```python
from build123d import *

# Parameters (mm, degrees)
SKETCH1_W               = 120
SKETCH1_H               = 220
BOSS_EXTRUDE1_DEPTH     = 50
SKETCH2_W               = 140
SKETCH2_H               = 240
BOSS_EXTRUDE2_DEPTH     = 1.5
SHELL1_T                = 2
CUT_EXTRUDE1_DEPTH      = 183.855817518
CUT_EXTRUDE1_DEPTH_BACK = 183.855817518
FILLET1_R               = 2
FILLET2_R               = 2
SKETCH9_R               = 4.951117386
CUT_EXTRUDE2_DEPTH      = 149.162917088
F_1_5MM_DOWEL_HOLE1_D   = 1.5


with BuildPart() as part:
    # Sketch1 → Boss-Extrude1 (new body)
    with BuildSketch(Plane.XY):
        Rectangle(SKETCH1_W, SKETCH1_H)
    extrude(amount=BOSS_EXTRUDE1_DEPTH)

    # Sketch2 → Boss-Extrude2 (add)
    with BuildSketch(Plane.XY.offset(50)):
        Rectangle(SKETCH2_W, SKETCH2_H)
    extrude(amount=BOSS_EXTRUDE2_DEPTH)

    # Shell1
    # the kernel refuses this shell: the inside is offset whole and opened at the faces by hand
    shell1_offset = offset(amount=-SHELL1_T, mode=Mode.PRIVATE)
    shell1_offset = shell1_offset + extrude(shell1_offset.faces().sort_by_distance((0, 0, 49.5))[0], amount=SHELL1_T, mode=Mode.PRIVATE)
    add(shell1_offset, mode=Mode.SUBTRACT)

    # Sketch8 → Cut-Extrude1 (cut, two sides: drawn at the far end of the back side and taken through both)
    with BuildSketch(Plane.ZY.offset(-58).offset(-CUT_EXTRUDE1_DEPTH_BACK)):
        with BuildLine():
            Line((51.5, -83), (44.5, -83))
            ThreePointArc((44.5, -83), (41, -86.5), (44.5, -90))
            Line((44.5, -90), (51.5, -90))
            Line((51.5, -90), (51.5, -83))
        make_face()
    extrude(amount=CUT_EXTRUDE1_DEPTH + CUT_EXTRUDE1_DEPTH_BACK, mode=Mode.SUBTRACT)

    # Fillet1
    fillet1_edges = [part.edges().sort_by_distance(p)[0] for p in [
        (0, -108, 2),
        (-60, 0, 0),
        (0, 110, 0),
        (60, 0, 0),
    ]]
    fillet(fillet1_edges, radius=FILLET1_R)

    # Fillet2
    # the kernel refuses this fillet: 2 mm, written as the material it adds along each edge
    with BuildSketch(Plane(origin=(58, 108, 51.5), x_dir=(0, -1, 0), z_dir=(0, 0, -1))) as fillet2_piece_1:
        with BuildLine():
            CenterArc((FILLET2_R, FILLET2_R), FILLET2_R, 180, 90)
            Line((0, FILLET2_R), (0, 0))
            Line((0, 0), (FILLET2_R, 0))
        make_face()
    extrude(amount=49.5)
    # the kernel refuses this fillet: 2 mm, written as the material it takes off along each edge
    with BuildSketch(Plane(origin=(-58, 108, 2), x_dir=(0, 1, 0), z_dir=(-1, 0, 0))) as fillet2_2_piece_1_section:
        Polygon((0, 0), (FILLET2_R * 1.02, 0), (FILLET2_R * 1.02, FILLET2_R * 1.02), (0, FILLET2_R * 1.02), align=None)
    fillet2_2_piece_1 = extrude(amount=FILLET2_R * 1.02, mode=Mode.PRIVATE)
    fillet2_2_piece_1 = fillet2_2_piece_1 - Plane(origin=(-58, 108, 2), x_dir=(0, -0.7071067811865475, 0.7071067811865475), z_dir=(-1, 0, 0)) * Sphere(FILLET2_R, mode=Mode.PRIVATE)
    add(fillet2_2_piece_1, mode=Mode.SUBTRACT)
    with BuildSketch(Plane(origin=(60, -110, 2), x_dir=(-1, 0, 0), z_dir=(0, 0, 1)), Plane(origin=(-60, -110, 2), x_dir=(0, 1, 0), z_dir=(0, 0, 1))) as fillet2_2_piece_2:
        with BuildLine():
            CenterArc((FILLET2_R, -FILLET2_R), FILLET2_R, 90, 90)
            Line((0, -FILLET2_R), (0, 0))
            Line((0, 0), (FILLET2_R, 0))
        make_face()
    extrude(amount=48, mode=Mode.SUBTRACT)
    with BuildSketch(Plane(origin=(-60, 110, 2), x_dir=(0, -1, 0), z_dir=(0, 0, 1))) as fillet2_2_piece_3:
        with BuildLine():
            CenterArc((FILLET2_R, FILLET2_R), FILLET2_R, 180, 90)
            Line((0, FILLET2_R), (0, 0))
            Line((0, 0), (FILLET2_R, 0))
        make_face()
    extrude(amount=48, mode=Mode.SUBTRACT)
    with BuildSketch(Plane(origin=(58, -110, 0), x_dir=(0, 0, 1), z_dir=(-1, 0, 0))) as fillet2_2_piece_4:
        with BuildLine():
            CenterArc((FILLET2_R, FILLET2_R), FILLET2_R, 180, 90)
            Line((0, FILLET2_R), (0, 0))
            Line((0, 0), (FILLET2_R, 0))
        make_face()
    extrude(amount=116, mode=Mode.SUBTRACT)
    with BuildSketch(Plane(origin=(58, -110, 2), x_dir=(1, 0, 0), z_dir=(0, 0, 1))) as fillet2_2_piece_5:
        with BuildLine():
            CenterArc((2 - FILLET2_R, FILLET2_R), FILLET2_R, 270, 90)
            Line((2, FILLET2_R), (2, 0))
            Line((2, 0), (2 - FILLET2_R, 0))
        make_face()
    revolve(axis=Axis((58, -110, 2), (0, 1, 0)), revolution_arc=90, mode=Mode.SUBTRACT)
    with BuildSketch(Plane(origin=(-58, -110, 2), x_dir=(-1, 0, 0), z_dir=(0, 0, 1))) as fillet2_2_piece_6:
        with BuildLine():
            CenterArc((2 - FILLET2_R, -FILLET2_R), FILLET2_R, 0, 90)
            Line((2 - FILLET2_R, 0), (2, 0))
            Line((2, 0), (2, -FILLET2_R))
        make_face()
    revolve(axis=Axis((-58, -110, 2), (0, -1, 0)), revolution_arc=90, mode=Mode.SUBTRACT)

    # Sketch9 → Cut-Extrude2 (cut, through all)
    with BuildSketch(Plane(origin=(0, 0, 0), x_dir=(-1, 0, 0), z_dir=(0, 0, -1))):
        with Locations((0, -88)):
            Circle(SKETCH9_R)
    extrude(amount=-CUT_EXTRUDE2_DEPTH, mode=Mode.SUBTRACT)

    # Ø1.5mm Dowel Hole1 (through all)
    with Locations(Plane(origin=(-164.627139737, -264.125226739, 50), x_dir=(-1, 0, 0), z_dir=(0, 0, -1))):
        with Locations((-229.627139737, 379.125226739), (-99.627139737, 379.125226739), (-229.627139737, 149.125226739), (-99.627139737, 149.125226739)):
            Hole(F_1_5MM_DOWEL_HOLE1_D / 2)


solid = part.part
```
Geometry check sheet. Reference: the model listing, model coordinates, mm. A direction names the side the tool comes from. Round coordinates to 2 decimals unless told otherwise and drop trailing zeros. Loops run counter-clockwise (first coordinate to the right, second up) from the corner with the lowest first, then second, coordinate; pieces in that order, holes last. Notation, with made-up numbers: (49.5, -38.5) - (64.5, -38.5) arc R15 ccw to (64.5, -27.5) - close; hole circle Ø1 at (48.5, 44.5). An arc over 180 degrees is marked (long way). Write each question's results on one line, items separated by ' | '. Start each with the question number.
Q1. Access from +Z, -Z, +X, -X, +Y, -Y to the whole of each face (thin tool, end or side, straight path). Record for faces 4 (the flat face through (-1, -110, 26)), 5 (the flat face through (-60, -2, 26)), 6 (the flat face through (-63, 34, 50)).
Q2. Cross-section at A-A on x = 0. Enter the section's corners in (y, z), and give its area (3 significant figures).
Q3. Thickness scan on line 1 (X direction, y = -115, z = 50.55); line 2 (Y direction, x = 65, z = 50.65); line 3 (X direction, y = -6, z = 32). Record the ranges inside material, lowest first. Write a range as [from, to].
Q4. Cross-section at B-B on z = 47. Enter the section's corners in (x, y), and give its area (3 significant figures).
Q5. Cross-section at D-D on y = 58. Enter the section's corners in (x, z).
Q6. Cross-section at C-C on z = 15. Enter the section's corners in (x, y), and give its area (3 significant figures).
Q7. Gauge pin test, flat ends, axial feed: P1, Ø2, axis at x = 65, y = 115, coming from the -Z side; P2, Ø10, axis at x = 40.5, z = 29.5, coming from the -Y side; P3, Ø1, axis at x = -55, y = 6, coming from the +Z side; P4, Ø0.9, axis at x = -65, y = 115, coming from the -Z side. Record the tip position at first contact, or that the pin passes through.
Q8. Release check for a two-part mould opening along X. For faces 1 (the flat face through (60, -1, 26)), 2 (the flat face through (-1, -108, 27)), 3 (the flat face through (62, 41, 51.5)) record: +X half, -X half, draft (parallel to the pull), parting line (faces both ways), or undercut.
Answers below:
1) face 4: -Z, +X, -X, -Y | face 5: -Z, -X, +Y, -Y | face 6: -Z, +Y
2) outline: (-120, 50) - (-110, 50) - (-110, 2) arc R2 ccw to (-108, 0) - (-92.95, 0) - (-92.95, 2) - (-106, 2) arc R2 cw to (-108, 4) - (-108, 51.5) - (-120, 51.5) - close; (-83.05, 0) - (108, 0) arc R2 ccw to (110, 2) - (110, 50) - (120, 50) - (120, 51.5) - (108, 51.5) - (108, 2) - (-83.05, 2) - close | area: 647 mm²
3) line 1: x = [-70, -65.75], [-64.25, 64.25], [65.75, 70] | line 2: y = [-120, -115.75], [-114.25, -90], [-83, 114.25], [115.75, 120] | line 3: x = [-60, -58], [58, 60]
4) outline: (-60, -108) arc R2 ccw to (-58, -110) - (58, -110) arc R2 ccw to (60, -108) - (60, -90) - (58, -90) - (58, -108) - (-58, -108) - (-58, -90) - (-60, -90) - close; (-60, -83) - (-58, -83) - (-58, 108) - (56, 108) arc R2 cw to (58, 106) - (58, -83) - (60, -83) - (60, 110) - (-58, 110) arc R2 ccw to (-60, 108) - close | area: 1,310 mm²
5) outline: (-70, 50) - (-60, 50) - (-60, 2) arc R2 ccw to (-58, 0) - (58, 0) arc R2 ccw to (60, 2) - (60, 50) - (70, 50) - (70, 51.5) - (58, 51.5) - (58, 2) - (-58, 2) - (-58, 51.5) - (-70, 51.5) - close
6) outline: (-60, -108) arc R2 ccw to (-58, -110) - (58, -110) arc R2 ccw to (60, -108) - (60, 110) - (-58, 110) arc R2 ccw to (-60, 108) - close; hole (-58, -108) - (58, -108) - (58, 106) arc R2 ccw to (56, 108) - (-58, 108) - close | area: 1,340 mm²
7) P1: stops at z = 50 | P2: stops at y = -110 | P3: stops at z = 2 | P4: passes through
8) face 1: +X half | face 2: undercut | face 3: draft
